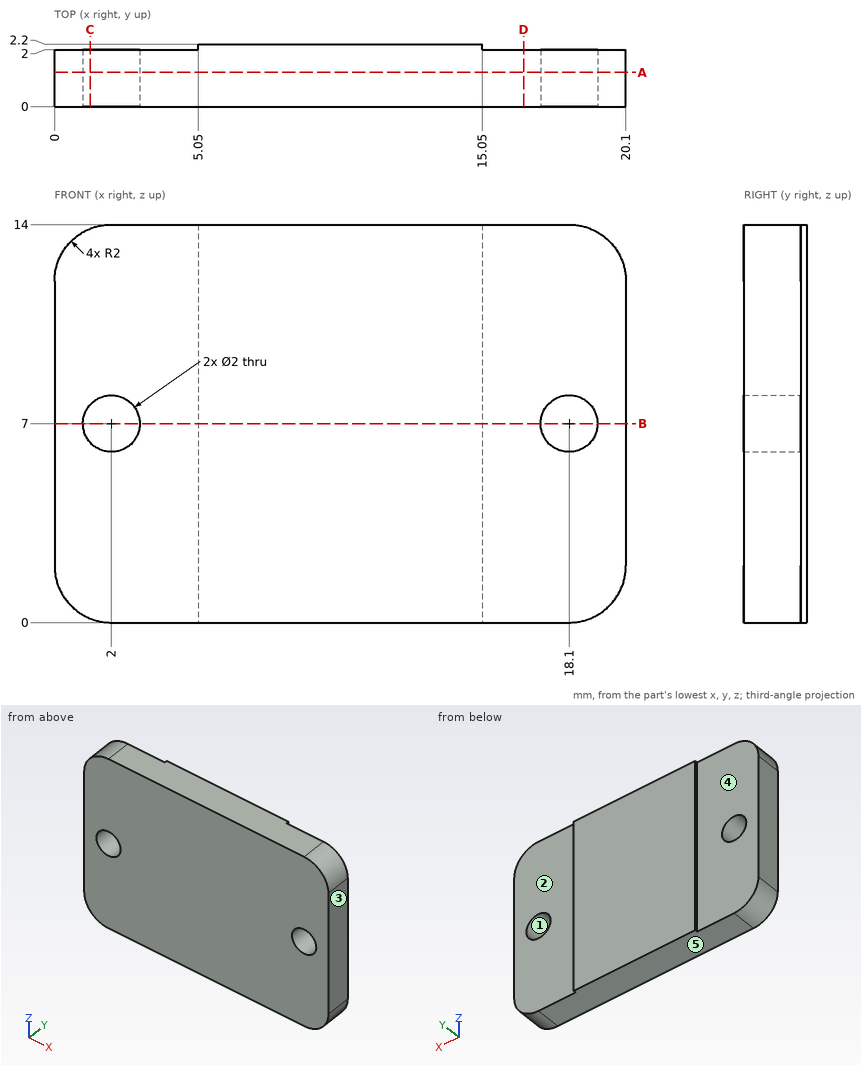
Verification items for this drawing (mm, ordinates from the low corner). A direction names the side the tool comes from. Coordinates: 2 decimals unless noted, no trailing zeros. Order: outer loops, then holes, each group sorted by start corner. A loop starts at its lowest first (then second) coordinate and runs counter-clockwise, first axis right, second up. Notation, with made-up numbers: (56.5, 14) -> (107.5, 14) arc R18 cw to (107.5, 42) -> close; hole circle Ø2 at (-25, 49). An arc over 180 degrees is marked (long way). Put each result on its own line as item: value. Start each with the question number.
1. Material ranges on L1, parallel to X at y = 1.25, z = 7; L2, parallel to Z at x = 18.1, y = 1.25; L3, parallel to Y at x = 18.75, z = 4, recorded low to high. Write a range as [from, to].
2. Mould release check, pull along X, two halves, no side actions. Record for the marked faces 1, 2 and 3: released by +X, released by -X, zero draft, split by the parting line, or undercut.
3. Cross-section at A-A, the plane y = 1.2. Record the boundary of the cut face in (x, z).
4. Cross-section at C-C, the plane x = 1.25. Record the boundary of the cut face in (y, z), then the cut area to 3 significant figures.
5. Go/stop test with flat-tipped pins: pin 1 Ø1.6 at (x, z) = (18.1, 7) entering from +Y; pin 2 Ø1.5 at (x, z) = (1.5, 6.5) entering from +Y; pin 3 Ø2.5 at (x, z) = (2, 7) entering from -Y. Record where each tip stops, or that it passes through.
6. Access from +Z, -Z, +X, -X, +Y, -Y to the whole of each face (thin tool, end or side, straight path). Record for the marked faces 4 and 5.
7. Cross-section at B-B, the plane z = 7. Record the boundary of the cut face in (x, y).
8. Cross-section at D-D, the plane x = 16.5. Record the boundary of the cut face in (y, z).
Computed:
1. L1: [0, 1], [3, 17.1], [19.1, 20.1]
1. L2: [0, 6], [8, 14]
1. L3: [0, 2]
2. face 1: undercut
2. face 2: zero draft
2. face 3: released by +X
3. outline: (0, 2) arc R2 ccw to (2, 0) -> (18.1, 0) arc R2 ccw to (20.1, 2) -> (20.1, 12) arc R2 ccw to (18.1, 14) -> (2, 14) arc R2 ccw to (0, 12) -> close; hole circle Ø2 at (2, 7); hole circle Ø2 at (18.1, 7)
4. outline: (0, 0.15) -> (2, 0.15) -> (2, 6.34) -> (0, 6.34) -> close; (0, 7.66) -> (2, 7.66) -> (2, 13.85) -> (0, 13.85) -> close
4. area: 24.8 mm2
5. pin 1: through
5. pin 2: y = 2
5. pin 3: y = 0
6. face 4: +Z, -Z, -X, +Y
6. face 5: -Z, +X, -X, +Y, -Y
7. outline: (0, 0) -> (1, 0) -> (1, 2) -> (0, 2) -> close; (3, 0) -> (17.1, 0) -> (17.1, 2) -> (15.05, 2) -> (15.05, 2.2) -> (5.05, 2.2) -> (5.05, 2) -> (3, 2) -> close; (19.1, 0) -> (20.1, 0) -> (20.1, 2) -> (19.1, 2) -> close
8. outline: (0, 0) -> (2, 0) -> (2, 14) -> (0, 14) -> close
